Solid Edge part; units mm, degrees
sketch "Sketch1" plane through (0, 0, 0) normal (0, 0, 1) x (1, 0, 0)
  line L0 (-6, -8) -> (6, -8)
  line L1 (6, -8) -> (6, 8)
  line L2 (6, 8) -> (-6, 8)
  line L3 (-6, 8) -> (-6, -8)
  circle A0 centre (0, 0) radius 1.7
extrude "Protrusion1" add sketch "Sketch1" along normal blind 50
Design review of the part built by this model. Coordinates are the model's own, in mm. Give positions to 0.01 mm unless a question says otherwise; leave off trailing zeros. Loops run counter-clockwise (first coordinate to the right, second up) from the corner with the lowest first, then second, coordinate; pieces in that order, holes last. Notation, with made-up numbers: M 63,15.25 L 86,15.25 A13 cw 86,26.25 Z; hole C -8,41.25 d1. An arc over 180 degrees is marked long. Answer as a JSON object with one key per item and string values.
Item 1: We need section A-A (y = 0). State the section outline as (x, z) points, and give its area (3 significant figures).
Output values:
{"outline": "M -6,0 L -1.7,0 L -1.7,50 L -6,50 Z; M 1.7,0 L 6,0 L 6,50 L 1.7,50 Z", "area": "430 mm2"}
Item 2: Mouldability with a two-part tool opening along X and no side actions: class faces 1 (the face through (-6, 0, 25)), 2 (the face through (0, -8, 25)), 3 (the face through (-0.37, 1.66, 24.65)), 4 (the face through (6, 0, 25)) as pulls with the +X half, pulls with the -X half, needs draft (parallel to the pull), parting line crosses it, or undercut.
Output values:
{"face 1": "pulls with the -X half", "face 2": "needs draft", "face 3": "undercut", "face 4": "pulls with the +X half"}
Item 3: We need section B-B (x = 0). State the section outline as (y, z) points.
Output values:
{"outline": "M -8,0 L -1.7,0 L -1.7,50 L -8,50 Z; M 1.7,0 L 8,0 L 8,50 L 1.7,50 Z"}
Item 4: We need section C-C (z = 44). State the section outline as (x, y) points.
Output values:
{"outline": "M -6,-8 L 6,-8 L 6,8 L -6,8 Z; hole C 0,0 d3.4"}
Item 5: Wall thickness on line 1 along Y through (x, z) = (0, 34); line 2 along Y through (x, z) = (-1, 16); line 3 along X through (y, z) = (1.5, 37): over which ranges is each line inside the solid? List them lowest first.
Output values:
{"line 1": "y = -8 to -1.7, 1.7 to 8", "line 2": "y = -8 to -1.37, 1.37 to 8", "line 3": "x = -6 to -0.8, 0.8 to 6"}
